from build123d import *

# Parameters (mm, degrees)
SKETCH1_W           = 220
SKETCH1_H           = 30
SKETCH1_R           = 2
BOSS_EXTRUDE1_DEPTH = 4
FILLET1_R           = 10
SKETCH2_R           = 5
CUT_EXTRUDE1_DEPTH  = 10


with BuildPart() as part:
    # Sketch1 → Boss-Extrude1 (new body)
    with BuildSketch(Plane.XY):
        with Locations((-110, -15)):
            Rectangle(SKETCH1_W, SKETCH1_H)
        with Locations((-205, -15)):
            Circle(SKETCH1_R, mode=Mode.SUBTRACT)
        with Locations((-13.75, -16)):
            Circle(SKETCH1_R, mode=Mode.SUBTRACT)
    extrude(amount=BOSS_EXTRUDE1_DEPTH)

    # Fillet1
    fillet1_edges = [part.edges().sort_by_distance(p)[0] for p in [
        (0, -30, 2),
        (-220, -30, 2),
        (-220, 0, 2),
        (0, 0, 2),
    ]]
    fillet(fillet1_edges, radius=FILLET1_R)

    # Sketch2 → Cut-Extrude1 (cut)
    with BuildSketch(Plane.XY.offset(4)):
        with Locations((-185, -15)):
            Circle(SKETCH2_R)
        with Locations((-110, -15)):
            Circle(SKETCH2_R)
        with Locations((-35, -15)):
            Circle(SKETCH2_R)
    extrude(amount=-CUT_EXTRUDE1_DEPTH, mode=Mode.SUBTRACT)


solid = part.part
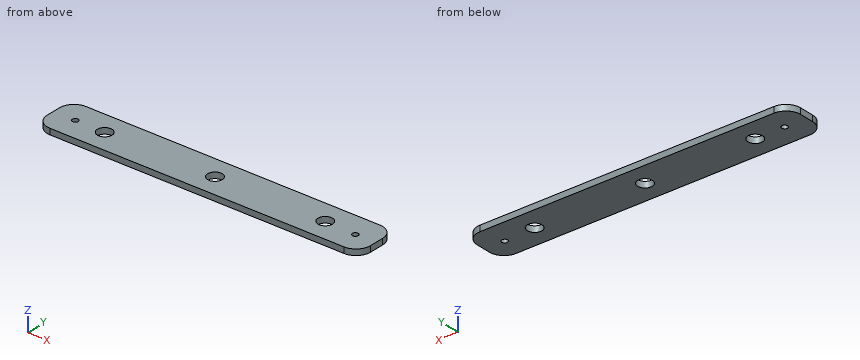
Geometry check sheet. Reference: the model listing, model coordinates, mm. Round coordinates to 2 decimals unless told otherwise and drop trailing zeros. Loops run counter-clockwise (first coordinate to the right, second up) from the corner with the lowest first, then second, coordinate; pieces in that order, holes last. Notation, with made-up numbers: (-3, -4) - (39, -4) arc R16 cw to (39, 12) - close; hole circle Ø9 at (27.5, 40). An arc over 180 degrees is marked (long way). One line per question, with ' | ' between items. Start each with the question number.
1. Depth check by flat-ended pin: pin 1 (11.5 mm diameter, centred on x = -35, y = -15, fed in from +Z); pin 2 (1 mm diameter, centred on x = -186, y = -19, fed in from +Z). Enter the tip coordinate at first touch or a pass-through.
2. Scan lines: line 1 (Y direction, x = -13.75, z = 0.85); line 2 (Y direction, x = -185, z = 2); line 3 (X direction, y = -18.5, z = 3.4). Record each from-to range of solid material in increasing order. Write a range as [from, to].
3. Cross-section at B-B on z = 0.9. Record the cut outline in (x, y).
4. Cross-section at C-C on x = -13.75. Record the cut outline in (y, z), then the cut area to 3 significant figures.
5. Cross-section at A-A on x = -185. Record the cut outline in (y, z).
6. Cross-section at D-D on y = -28. Record the cut outline in (x, z), then the cut area to 3 significant figures.
Taken from the geometry:
1) pin 1: z = 4 | pin 2: through
2) line 1: [-30, -18], [-14, 0] | line 2: [-30, -20], [-10, 0] | line 3: [-220, -188.57], [-181.43, -113.57], [-106.43, -38.57], [-31.43, 0]
3) outline: (-220, -20) arc R10 ccw to (-210, -30) - (-10, -30) arc R10 ccw to (0, -20) - (0, -10) arc R10 ccw to (-10, 0) - (-210, 0) arc R10 ccw to (-220, -10) - close; hole circle Ø4 at (-205, -15); hole circle Ø10 at (-185, -15); hole circle Ø10 at (-110, -15); hole circle Ø10 at (-35, -15); hole circle Ø4 at (-13.75, -16)
4) outline: (-30, 0) - (-18, 0) - (-18, 4) - (-30, 4) - close; (-14, 0) - (0, 0) - (0, 4) - (-14, 4) - close | area: 104 mm²
5) outline: (-30, 0) - (-20, 0) - (-20, 4) - (-30, 4) - close; (-10, 0) - (0, 0) - (0, 4) - (-10, 4) - close
6) outline: (-216, 0) - (-4, 0) - (-4, 4) - (-216, 4) - close | area: 848 mm²
